Input: part model. Units: mm. Frame: model coordinates. Face numbers are marked on the shaded views. A direction names the side the tool comes from. Coordinates: 2 decimals unless noted, no trailing zeros. Order: outer loops, then holes, each group sorted by start corner. A loop starts at its lowest first (then second) coordinate and runs counter-clockwise, first axis right, second up. Notation, with made-up numbers: (1.5, 18) - (44.5, 18) arc R29 cw to (44.5, 56) - close; hole circle Ø6 at (-5.75, 89). An arc over 180 degrees is marked (long way). Answer as CSV lines item,"result". Start each with the question number.
Item 1: Material intervals for line 1 along Y through (x, z) = (1.35, 0); line 2 along Y through (x, z) = (1.45, 0); line 3 along X through (y, z) = (-4.5, 2.25), sorted ascending.
Item 2: Draft query along Z for the marked faces 4, 5 and 6. Return one class per face: +Z half, -Z half, draft (parallel to the pull), parting line (faces both ways), or undercut.
Item 3: Section A-A (y = 0). State how many separate pieces and enclosed holes the cut face has, and give its area (3 significant figures).
Item 4: Section C-C (x = -0.5). Output: boundary loops of the cut face in (y, z), and give its area (3 significant figures).
Item 5: Section D-D (x = -2.05). Output: boundary loops of the cut face in (y, z).
Item 6: Access query for the marked faces 1, 2 and 3. Directions: +Z, -Z, +X, -X, +Y, -Y. A direction counts if a zero-diameter tool reaches every point of the face in a straight line with its end or side. Return the directions, or none.
Item 7: First-contact query: pin 1 (1 mm diameter, centred on x = 1, y = 2.5, fed in from -Z); pin 2 (4.5 mm diameter, centred on y = 0, z = 0, fed in from -X); pin 3 (1 mm diameter, centred on x = -0.5, y = 3.5, fed in from -Z). Flat tips, straight axial feed; report the tip coordinate or a pass-through.
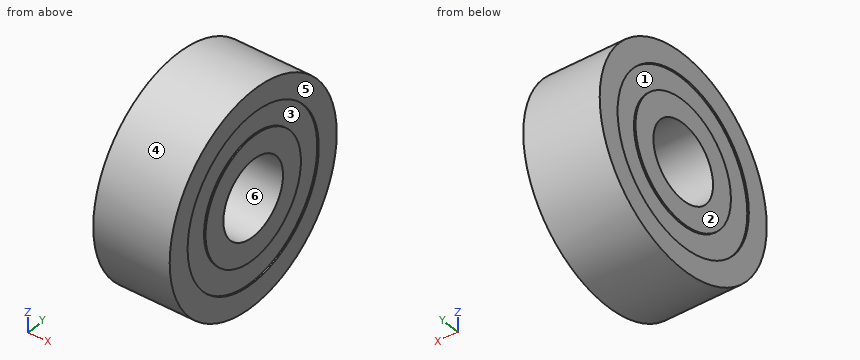
from build123d import *


with BuildPart() as part:
    # Sketch → Revolution (revolve)
    with BuildSketch(Plane.YX):
        Polygon((-7, 2.5), (-5.5, 2.5), (-5.5, 2.4), (-4, 2.4), (-4, 2.5), (-2.5, 2.5), (-2.5, -2.5), (-4, -2.5), (-4, -2.4), (-5.5, -2.4), (-5.5, -2.5), (-7, -2.5), align=None)
        with BuildLine():
            ThreePointArc((-5.5, 1.299038), (-6.25, 0), (-5.5, -1.299038))
            Line((-5.5, -1.299038), (-5.5, -1.4))
            Line((-4, -1.4), (-5.5, -1.4))
            Line((-4, -1.4), (-4, -1.299038))
            ThreePointArc((-4, -1.299038), (-3.25, 0), (-4, 1.299038))
            Line((-4, 1.299038), (-4, 1.4))
            Line((-5.5, 1.4), (-4, 1.4))
            Line((-5.5, 1.4), (-5.5, 1.299038))
        make_face(mode=Mode.SUBTRACT)
    revolve(axis=Axis((0, 0, 0), (1, 0, 0)))


solid = part.part
Determined:
1,line 1,"y = -7 to -5.5, -4 to -2.5, 2.5 to 4, 5.5 to 7"
1,line 2,"y = -7 to -2.5, 2.5 to 7"
1,line 3,"x = -2.4 to -1.4, 1.4 to 2.4"
2,face 4,"parting line"
2,face 5,"draft"
2,face 6,"undercut"
3,separate pieces,"2"
3,enclosed holes,"2"
3,area,"30.5 mm^2"
4,outline,"circle Ø14 at (0, 0); circle Ø6.67 at (0, 0); hole circle Ø12.33 at (0, 0); hole circle Ø5 at (0, 0)"
4,area,"49.9 mm^2"
5,outline,"circle Ø14 at (0, 0); hole circle Ø5 at (0, 0)"
6,face 1,"-X"
6,face 2,"+Z, -Z, -X, +Y, -Y"
6,face 3,"+X"
7,pin 1,"stops at z = -6.71"
7,pin 2,"passes through"
7,pin 3,"stops at z = -6.32"
